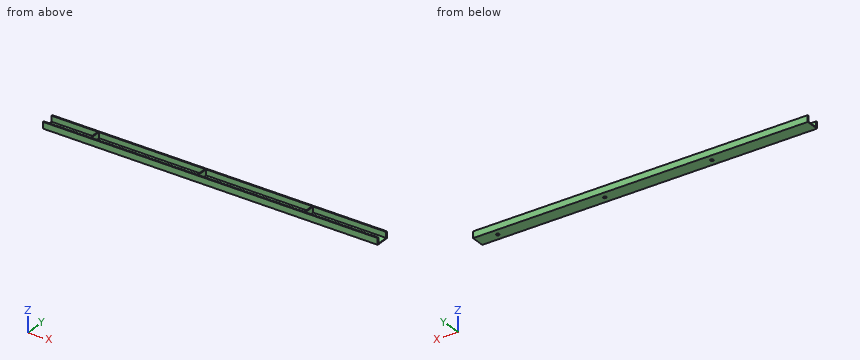
```python
from build123d import *

# Parameters (mm, degrees)
SKETCH_1_W             = 4300
SKETCH_1_H             = 100
EXTRUDE_1_DEPTH        = 48
SKETCH_2_W             = 4300
SKETCH_2_H             = 83
CUT_EXTRUDE_2_DEPTH    = 42.7
SKETCH_3_W             = 8.5
SKETCH_3_H             = 83
EXTRUDE_3_DEPTH        = 42.7
PATTERN_LINEAR_1_COUNT = 5
PATTERN_LINEAR_1_PITCH = 800
SKETCH_4_R             = 11.5
CUT_EXTRUDE_4_DEPTH    = 4302.430459742
PATTERN_LINEAR_2_COUNT = 6
PATTERN_LINEAR_2_PITCH = 800
SKETCH_5_W             = 1800
SKETCH_5_H             = 100
CUT_EXTRUDE_1_DEPTH    = 48


with BuildPart() as part:
    # 草图1 → 拉伸1 (new body)
    with BuildSketch(Plane.XY):
        with Locations((2150, 50)):
            Rectangle(SKETCH_1_W, SKETCH_1_H)
    extrude(amount=EXTRUDE_1_DEPTH)

    # 草图2 → 拉伸2 (cut)
    with BuildSketch(Plane.XY.offset(48)):
        with Locations((2150, 50)):
            Rectangle(SKETCH_2_W, SKETCH_2_H)
    extrude(amount=-CUT_EXTRUDE_2_DEPTH, mode=Mode.SUBTRACT)

    # 草图3 → 拉伸3 (add)
    with BuildSketch(Plane.XY.offset(5.3)):
        with Locations((550, 50)):
            Rectangle(SKETCH_3_W, SKETCH_3_H)
    extrude_3 = extrude(amount=EXTRUDE_3_DEPTH)

    # 阵列(线性)1: 拉伸3 ×5
    with Locations(*[(i * PATTERN_LINEAR_1_PITCH, 0, 0) for i in range(1, PATTERN_LINEAR_1_COUNT)]):
        add(extrude_3)

    # 草图4 → 拉伸4 (cut, through all)
    with BuildSketch(Plane(origin=(0, 0, 0), x_dir=(-1, 0, 0), z_dir=(0, 0, -1))):
        with Locations((-4150, 50)):
            Circle(SKETCH_4_R)
    cut_extrude_4 = extrude(amount=-CUT_EXTRUDE_4_DEPTH, mode=Mode.SUBTRACT)

    # 阵列(线性)2: 拉伸4 ×6
    with Locations(*[(-i * PATTERN_LINEAR_2_PITCH, 0, 0) for i in range(1, PATTERN_LINEAR_2_COUNT)]):
        add(cut_extrude_4, mode=Mode.SUBTRACT)

    # 草图5 → 切除-拉伸1 (cut)
    with BuildSketch(Plane(origin=(0, 0, 0), x_dir=(-1, 0, 0), z_dir=(0, 0, -1))):
        with Locations((-900, 50)):
            Rectangle(SKETCH_5_W, SKETCH_5_H)
    extrude(amount=-CUT_EXTRUDE_1_DEPTH, mode=Mode.SUBTRACT)


solid = part.part
```
Work out the finished part from the listing and answer in its coordinate system (mm). Give positions to 0.01 mm unless a question says otherwise; leave off trailing zeros. Loops run counter-clockwise (first coordinate to the right, second up) from the corner with the lowest first, then second, coordinate; pieces in that order, holes last. Notation, with made-up numbers: (40.5, 76.25) -> (81.5, 76.25) arc R28 ccw to (81.5, 103.25) -> close; hole circle Ø6 at (53, -32.5). An arc over 180 degrees is marked (long way). Use CSV: the item, a comma, the result in double quotes.
1. The part is cut by section A-A (z = 23.5). Write down the section's boundary in (x, y).
Found:
outline,"(1800, 0) -> (4300, 0) -> (4300, 8.5) -> (3754.25, 8.5) -> (3754.25, 91.5) -> (4300, 91.5) -> (4300, 100) -> (1800, 100) -> (1800, 91.5) -> (2145.75, 91.5) -> (2145.75, 8.5) -> (1800, 8.5) -> close; hole (2154.25, 8.5) -> (2945.75, 8.5) -> (2945.75, 91.5) -> (2154.25, 91.5) -> close; hole (2954.25, 8.5) -> (3745.75, 8.5) -> (3745.75, 91.5) -> (2954.25, 91.5) -> close"
2. The part is cut by section B-B (x = 2904). Write down the section's boundary in (y, z), then the cut area to 3 significant figures.
Found:
outline,"(0, 0) -> (100, 0) -> (100, 48) -> (91.5, 48) -> (91.5, 5.3) -> (8.5, 5.3) -> (8.5, 48) -> (0, 48) -> close"
area,"1,260 mm^2"
3. Straight lines are drawn through the part: line 1 (X direction, y = 42, z = 19); line 2 (Y direction, x = 4150, z = 3.2); line 3 (Y direction, x = 2136.5, z = 20.5). For each, find the intervals that lie inside material, in ascending order.
Found:
line 1,"2145.75 to 2154.25, 2945.75 to 2954.25, 3745.75 to 3754.25"
line 2,"0 to 38.5, 61.5 to 100"
line 3,"0 to 8.5, 91.5 to 100"
4. Flat-ended cylindrical pins translate along their axes: pin 1 Ø13 at (y, z) = (32, 20.5) entering from +X; pin 2 Ø4 at (y, z) = (23, 25) entering from -X; pin 3 Ø8 at (x, y) = (3694, 54.5) entering from +Z. Find the tip coordinate at first contact, or state that the pin passes through.
Found:
pin 1,"x = 3754.25"
pin 2,"x = 2145.75"
pin 3,"z = 5.3"
